```python
from build123d import *

# Parameters (mm, degrees)
BOSS_EXTRUDE1_DEPTH = 100


with BuildPart() as part:
    # Sketch1 → Boss-Extrude1 (new, symmetric)
    with BuildSketch(Plane.XY):
        with BuildLine():
            Line((-13.496435042, -1.5), (-13.496435042, 1.5))
            ThreePointArc((-13.496435042, 1.5), (-12.627675159, 3.673771087), (-10.5, 4.65))
            Line((-10.5, 4.65), (10.5, 5.7))
            ThreePointArc((10.5, 5.7), (16.492120552, 0), (10.5, -5.7))
            Line((10.5, -5.7), (-10.5, -4.65))
            ThreePointArc((-10.5, -4.65), (-12.627675159, -3.673771087), (-13.496435042, -1.5))
        make_face()
    extrude(amount=BOSS_EXTRUDE1_DEPTH, both=True)


solid = part.part
```
Can you work these out from the model? Positions are in its coordinate system, mm. Give positions to 0.01 mm unless a question says otherwise; leave off trailing zeros. Loops run counter-clockwise (first coordinate to the right, second up) from the corner with the lowest first, then second, coordinate; pieces in that order, holes last. Notation, with made-up numbers: M 36,77.5 L 62,77.5 A23 cw 62,95.5 Z; hole C 5,33.5 d1. An arc over 180 degrees is marked long. Use one line per item in the form item = value. Start each with the question number.
(1) I want a section at C-C, the plane x = 12.25. Write out the boundary of the cut face in (y, z), and give its area (3 significant figures).
(2) I'm going to push flat-ended pins straight in: P1, Ø8, axis at x = -8.5, z = 69, coming from the -Y side; P2, Ø5, axis at x = 9.5, z = -15.5, coming from the -Y side; P3, Ø10, axis at x = 3, z = -65.5, coming from the -Y side (3 decimals). Where does each tip first touch, or does it pass through?
(3) Please list where these lines run through material, in increasing order: line 1 (Y direction, x = 11.5, z = 29); line 2 (X direction, y = -2.75, z = 19.5); line 3 (X direction, y = 1.5, z = 38).
(4) I want a section at A-A, the plane x = -8.5. Write out the boundary of the cut face in (y, z), and give its area (3 significant figures).
Worked out:
q1.outline = M -5.52,-100 L 5.52,-100 L 5.52,100 L -5.52,100 Z
q1.area = 2,210 mm²
q2.P1 = -4.95
q2.P2 = -5.71
q2.P3 = -5.575
q3.line_1 = -5.66 to 5.66
q3.line_2 = -13.24 to 15.79
q3.line_3 = -13.5 to 16.29
q4.outline = M -4.75,-100 L 4.75,-100 L 4.75,100 L -4.75,100 Z
q4.area = 1,900 mm²
